```python
from build123d import *

# Parameters (mm, degrees)
SKETCH1_W           = 60.325
SKETCH1_H           = 50.8
SKETCH1_R           = 2.4892
SKETCH1_R_2         = 2.5527
SKETCH1_R_3         = 14.2875
BOSS_EXTRUDE1_DEPTH = 6.35
FILLET1_R           = 6.35


with BuildPart() as part:
    # Sketch1 → Boss-Extrude1 (new body)
    with BuildSketch(Plane.XY):
        Rectangle(SKETCH1_W, SKETCH1_H)
        with Locations((-9.525, -19.05)):
            Circle(SKETCH1_R, mode=Mode.SUBTRACT)
        with Locations((9.525, -19.05)):
            Circle(SKETCH1_R, mode=Mode.SUBTRACT)
        with Locations((9.525, 19.05)):
            Circle(SKETCH1_R, mode=Mode.SUBTRACT)
        with Locations((-9.525, 19.05)):
            Circle(SKETCH1_R, mode=Mode.SUBTRACT)
        with Locations((22.225, 0)):
            Circle(SKETCH1_R, mode=Mode.SUBTRACT)
        with Locations((-22.225, 0)):
            Circle(SKETCH1_R, mode=Mode.SUBTRACT)
        with Locations((-19.731795339, -15.994256867)):
            Circle(SKETCH1_R_2, mode=Mode.SUBTRACT)
        with Locations((19.731795339, 15.994256867)):
            Circle(SKETCH1_R_2, mode=Mode.SUBTRACT)
        Circle(SKETCH1_R_3, mode=Mode.SUBTRACT)
    extrude(amount=BOSS_EXTRUDE1_DEPTH)

    # Fillet1
    fillet1_edges = [part.edges().sort_by_distance(p)[0] for p in [
        (30.1625, -25.4, 3.175),
        (-30.1625, -25.4, 3.175),
        (-30.1625, 25.4, 3.175),
        (30.1625, 25.4, 3.175),
    ]]
    fillet(fillet1_edges, radius=FILLET1_R)


solid = part.part
```
Source: CAD feature listing. Evaluate the final solid. Frame: model axes, mm. Give positions to 0.01 mm unless a question says otherwise; leave off trailing zeros. Loops run counter-clockwise (first coordinate to the right, second up) from the corner with the lowest first, then second, coordinate; pieces in that order, holes last. Notation, with made-up numbers: M 60.25,34 L 65.25,34 A31 cw 65.25,58 Z; hole C 12.25,-14 d10. An arc over 180 degrees is marked long. Put each result on its own line as item: value.
Q1. Section C-C (z = 5.5). Count the separate pieces of the cut face and the enclosed holes in it, and give its area (3 significant figures).
Response values:
separate pieces: 1
enclosed holes: 9
area: 2,230 mm²
Q2. Line query: probe 1 along Y at (x, z) = (0.5, 0.5); probe 2 along X at (y, z) = (1.5, 3.75); probe 3 along Y at (x, z) = (8, 1.25). Output: solid intervals per line, ascending. Write a range as [from, to].
Response values:
probe 1: y = [-25.4, -14.28], [14.28, 25.4]
probe 2: x = [-30.16, -24.21], [-20.24, -14.21], [14.21, 20.24], [24.21, 30.16]
probe 3: y = [-25.4, -21.02], [-17.08, -11.84], [11.84, 17.08], [21.02, 25.4]
Q3. Section D-D (y = 10). Return the cut outline in (x, z), and give its area (3 significant figures).
Response values:
outline: M -30.16,0 L -10.2,0 L -10.2,6.35 L -30.16,6.35 Z; M 10.2,0 L 30.16,0 L 30.16,6.35 L 10.2,6.35 Z
area: 253 mm²
Q4. Mould query, pull axis X, two halves, no side actions, for faces 1 (the cylindrical face through (-19.85, 0.75, 3.13)), 2 (the cylindrical face through (-28.35, -23.49, 3.22)), 3 (the flat face through (30.162, 0, 3)). Classes: released by +X, released by -X, zero draft, split by the parting line, or undercut.
Response values:
face 1: undercut
face 2: released by -X
face 3: released by +X
Q5. Section B-B (y = 0). Return the cut outline in (x, z), and give its area (3 significant figures).
Response values:
outline: M -30.16,0 L -24.71,0 L -24.71,6.35 L -30.16,6.35 Z; M -19.74,0 L -14.29,0 L -14.29,6.35 L -19.74,6.35 Z; M 14.29,0 L 19.74,0 L 19.74,6.35 L 14.29,6.35 Z; M 24.71,0 L 30.16,0 L 30.16,6.35 L 24.71,6.35 Z
area: 138 mm²
Q6. Section A-A (x = 0). Return the cut outline in (y, z).
Response values:
outline: M -25.4,0 L -14.29,0 L -14.29,6.35 L -25.4,6.35 Z; M 14.29,0 L 25.4,0 L 25.4,6.35 L 14.29,6.35 Z
